Part model, mm, in its own coordinate system. Give positions to 0.01 mm unless a question says otherwise; leave off trailing zeros. Answer as a JSON object with one key per item and string values. Group by question number.
```python
from build123d import *

# Parameters (mm, degrees)
SKETCH1_W           = 680
SKETCH1_H           = 50
SKETCH1_R           = 5
BOSS_EXTRUDE1_DEPTH = 23


with BuildPart() as part:
    # Sketch1 → Boss-Extrude1 (new body)
    with BuildSketch(Plane(origin=(0, 0, 0), x_dir=(0, 0, -1), z_dir=(1, 0, 0))):
        Rectangle(SKETCH1_W, SKETCH1_H)
        with Locations((-320, 0)):
            Circle(SKETCH1_R, mode=Mode.SUBTRACT)
        with Locations((-300, 0)):
            Circle(SKETCH1_R, mode=Mode.SUBTRACT)
        with Locations((-280, 0)):
            Circle(SKETCH1_R, mode=Mode.SUBTRACT)
        with Locations((-260, 0)):
            Circle(SKETCH1_R, mode=Mode.SUBTRACT)
        with Locations((-240, 0)):
            Circle(SKETCH1_R, mode=Mode.SUBTRACT)
        with Locations((-220, 0)):
            Circle(SKETCH1_R, mode=Mode.SUBTRACT)
        with Locations((-200, 0)):
            Circle(SKETCH1_R, mode=Mode.SUBTRACT)
        with Locations((-180, 0)):
            Circle(SKETCH1_R, mode=Mode.SUBTRACT)
        with Locations((-160, 0)):
            Circle(SKETCH1_R, mode=Mode.SUBTRACT)
        with Locations((-140, 0)):
            Circle(SKETCH1_R, mode=Mode.SUBTRACT)
        with Locations((-120, 0)):
            Circle(SKETCH1_R, mode=Mode.SUBTRACT)
        with Locations((-100, 0)):
            Circle(SKETCH1_R, mode=Mode.SUBTRACT)
        with Locations((-80, 0)):
            Circle(SKETCH1_R, mode=Mode.SUBTRACT)
        with Locations((-60, 0)):
            Circle(SKETCH1_R, mode=Mode.SUBTRACT)
        with Locations((-40, 0)):
            Circle(SKETCH1_R, mode=Mode.SUBTRACT)
        with Locations((-20, 0)):
            Circle(SKETCH1_R, mode=Mode.SUBTRACT)
        Circle(SKETCH1_R, mode=Mode.SUBTRACT)
        with Locations((20, 0)):
            Circle(SKETCH1_R, mode=Mode.SUBTRACT)
        with Locations((40, 0)):
            Circle(SKETCH1_R, mode=Mode.SUBTRACT)
        with Locations((60, 0)):
            Circle(SKETCH1_R, mode=Mode.SUBTRACT)
    extrude(amount=BOSS_EXTRUDE1_DEPTH)


solid = part.part
```
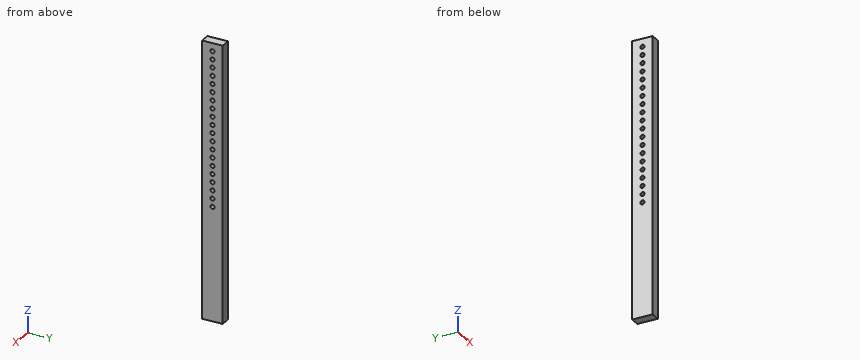
1) Band-saw the part on A-A (x = 10.5). State how many separate pieces and enclosed holes the cut face has, plus the area to 3 significant figures.
2) Probe line 1 (Y direction, x = 16.5, z = 260); line 2 (Y direction, x = 19.5, z = 61). List the from-to ranges inside material, lowest first.
3) Drop a flat-ended pin along its axis: P1, Ø9, axis at y = 0, z = 0, coming from the -X side. Give the stop position or say it passes through.
Verdict:
{
 "1": {"separate pieces": "1", "enclosed holes": "20", "area": "32,400 mm2"},
 "2": {"line 1": "-25 to -5, 5 to 25", "line 2": "-25 to -4.9, 4.9 to 25"},
 "3": {"P1": "through"}
}
